```python
from build123d import *

# Parameters (mm, degrees)
SKETCH1_R               = 1.5
BOSS_EXTRUDE1_DEPTH     = 5
CUT_EXTRUDE1_REACH      = 48.103
CUT_EXTRUDE1_END_RADIUS = 6.5
SKETCH2_R               = 2


with BuildPart() as part:
    # Sketch1 → Boss-Extrude1 (new body)
    with BuildSketch(Plane(origin=(0, 0, 0), x_dir=(0, 0, -1), z_dir=(1, 0, 0))):
        with BuildLine():
            Line((-5.5, 20), (-5.5, -20))
            Line((-5.5, -20), (5.5, -20))
            Line((5.5, -20), (5.5, 20))
            ThreePointArc((5.5, 20), (0, 25.5), (-5.5, 20))
        make_face()
        with Locations((0, 20)):
            Circle(SKETCH1_R, mode=Mode.SUBTRACT)
    extrude(amount=BOSS_EXTRUDE1_DEPTH)

    # Cut-Extrude1: up to this cylinder (the profile starts outside it)
    cut_extrude1_end = Plane(origin=(2.5, 20, 0), z_dir=(-1, 0, 0)) * Cylinder(CUT_EXTRUDE1_END_RADIUS, 110.206, mode=Mode.PRIVATE)
    # Sketch2 → Cut-Extrude1 (cut, up to the surface)
    with BuildSketch(Plane.XZ.offset(20), mode=Mode.PRIVATE) as cut_extrude1_sk1:
        with Locations(Location((2.5, 0, 0), (0, 0, 270))):
            Circle(SKETCH2_R)
    cut_extrude1_tool1 = extrude(cut_extrude1_sk1.sketch, amount=-CUT_EXTRUDE1_REACH, mode=Mode.PRIVATE) - cut_extrude1_end
    add(cut_extrude1_tool1.solids().sort_by_distance((2.5, -20, 0))[0], mode=Mode.SUBTRACT)


solid = part.part
```
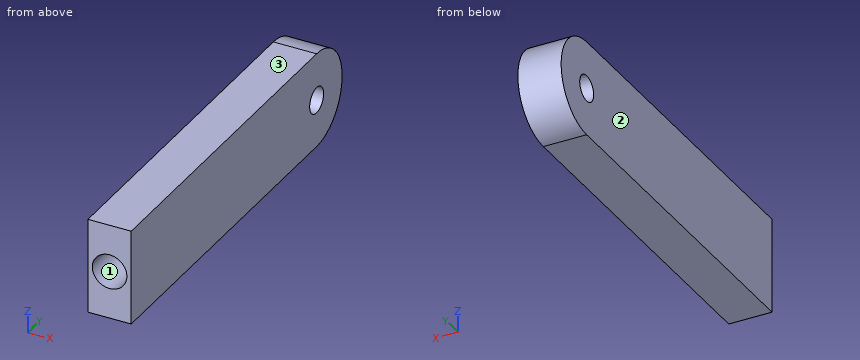
Source: CAD feature listing. Evaluate the final solid. Frame: model axes, mm. Face numbers are marked on the shaded views. Round coordinates to 2 decimals unless told otherwise and drop trailing zeros. Loops run counter-clockwise (first coordinate to the right, second up) from the corner with the lowest first, then second, coordinate; pieces in that order, holes last.
(1) Material intervals for probe 1 along X at (y, z) = (0.5, 0); probe 2 along Y at (x, z) = (2.65, 0); probe 3 along Z at (x, y) = (2.5, -9), sorted ascending.
From the geometry:
probe 1: x = 0 to 0.5, 4.5 to 5
probe 2: y = 13.5 to 18.5, 21.5 to 25.5
probe 3: z = -5.5 to -2, 2 to 5.5
(2) Pull-direction query (X, two-part tool) for the marked faces 1, 2 and 3; classes: +X half, -X half, draft (parallel to the pull), parting line (faces both ways), or undercut.
From the geometry:
face 1: undercut
face 2: -X half
face 3: draft
(3) Section query B-B (x = 2.5). Output: boundary loops of the cut face in (y, z).
From the geometry:
outline: (-20, -5.5) - (20, -5.5) arc R5.5 ccw to (20, 5.5) - (-20, 5.5) - (-20, 2) - (13.82, 2) arc R6.5 ccw to (13.82, -2) - (-20, -2) - close; hole circle Ø3 at (20, 0)
(4) Section query A-A (z = 0). Output: boundary loops of the cut face in (x, y).
From the geometry:
outline: (0, -20) - (0.5, -20) - (0.5, 13.5) - (4.5, 13.5) - (4.5, -20) - (5, -20) - (5, 18.5) - (0, 18.5) - close; (0, 21.5) - (5, 21.5) - (5, 25.5) - (0, 25.5) - close
(5) Section query C-C (y = -0.5). Output: boundary loops of the cut face in (x, z).
From the geometry:
outline: (0, -5.5) - (5, -5.5) - (5, 5.5) - (0, 5.5) - close; hole circle Ø4 at (2.5, 0)
(6) Section query D-D (z = -3). Output: boundary loops of the cut face in (x, y).
From the geometry:
outline: (0, -20) - (5, -20) - (5, 24.61) - (0, 24.61) - close
